Design review of the part built by this model. Coordinates are the model's own, in mm. Face numbers are marked on the shaded views. A direction names the side the tool comes from. Coordinates: 2 decimals unless noted, no trailing zeros. Write each loop counter-clockwise with the first axis right and the second up, starting at its lowest first coordinate (ties: lowest second). Pieces come first, ordered by that corner, then holes. Notation, with made-up numbers: (78.25, 5.5) - (100.25, 5.5) arc R13 ccw to (100.25, 14.5) - close; hole circle Ø8 at (80.25, 83.25). An arc over 180 degrees is marked (long way). Answer as a JSON object with one key per item and string values.
```python
from build123d import *

# Parameters (mm, degrees)
SKETCH1_R           = 6.65
BOSS_EXTRUDE1_DEPTH = 30
SKETCH2_W           = 8
SKETCH2_H           = 40
CUT_EXTRUDE1_DEPTH  = 70.462219947
FILLET1_R           = 4


with BuildPart() as part:
    # Sketch1 → Boss-Extrude1 (new body)
    with BuildSketch(Plane.XY):
        with BuildLine():
            Line((0, 0), (30, 0))
            Line((30, 0), (30, 40))
            ThreePointArc((30, 40), (15, 55), (0, 40))
            Line((0, 40), (0, 0))
        make_face()
        with Locations((15, 40)):
            Circle(SKETCH1_R, mode=Mode.SUBTRACT)
    extrude(amount=BOSS_EXTRUDE1_DEPTH)

    # Sketch2 → Cut-Extrude1 (cut, through all)
    with BuildSketch(Plane.ZY):
        with Locations((15, 35)):
            Rectangle(SKETCH2_W, SKETCH2_H)
    extrude(amount=-CUT_EXTRUDE1_DEPTH, mode=Mode.SUBTRACT)

    # Fillet1
    fillet1_edges = [part.edges().sort_by_distance(p)[0] for p in [
        (15, 15, 19),
        (15, 15, 11),
    ]]
    fillet(fillet1_edges, radius=FILLET1_R - 0.0001)  # a hair under: the kernel refuses the full size


solid = part.part
```
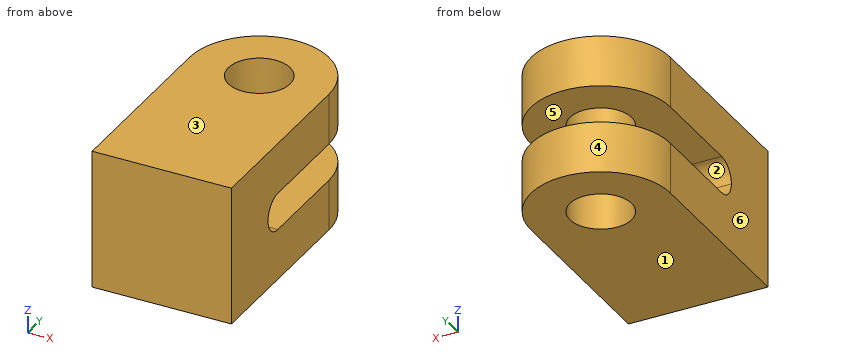
(1) For pin 1 (1 mm diameter, centred on x = 6, z = 24.5, fed in from +Y), flat-tipped, find the tip position at first contact; note if it passes through.
Solved:
{"pin 1": "stops at y = 52.36"}
(2) Take a section at A-A, the plane x = 15. Give the number of separate pieces and of enclosed holes in the cut face, and give its area (3 significant figures).
Solved:
{"separate pieces": "3", "enclosed holes": "0", "area": "1,040 mm^2"}
(3) Take a section at B-B, the plane y = 29.5. Write out the cut boundary in (x, z), and give its area (3 significant figures).
Solved:
{"outline": "(0, 0) - (30, 0) - (30, 11) - (0, 11) - close; (0, 19) - (30, 19) - (30, 30) - (0, 30) - close", "area": "660 mm^2"}
(4) Take a section at D-D, the plane y = 45. Write out the cut boundary in (x, z).
Solved:
{"outline": "(0.86, 0) - (10.62, 0) - (10.62, 11) - (0.86, 11) - close; (0.86, 19) - (10.62, 19) - (10.62, 30) - (0.86, 30) - close; (19.38, 0) - (29.14, 0) - (29.14, 11) - (19.38, 11) - close; (19.38, 19) - (29.14, 19) - (29.14, 30) - (19.38, 30) - close"}
(5) To check wall thickness, follow line 1 (Y direction, x = 15, z = 22.75); line 2 (Z direction, x = 16.75, y = 25.5); line 3 (X direction, y = 40, z = 3). State the ranges of each line that lie inside material, in increasing order. Write a range as from..to.
Solved:
{"line 1": "y = 0..33.35, 46.65..55", "line 2": "z = 0..11, 19..30", "line 3": "x = 0..8.35, 21.65..30"}
(6) Take a section at C-C, the plane z = 8. Write out the cut boundary in (x, y), and give its area (3 significant figures).
Solved:
{"outline": "(0, 0) - (30, 0) - (30, 40) arc R15 ccw to (0, 40) - close; hole circle Ø13.3 at (15, 40)", "area": "1,410 mm^2"}
(7) Tool access review of the marked faces 5 and 6: name each direction out of +Z, -Z, +X, -X, +Y, -Y from which nothing blocks a thin tool from reaching the whole face with its end or side.
Solved:
{"face 5": "+X, -X, +Y", "face 6": "+Z, -Z, -X, +Y, -Y"}
(8) The part is to be moulded in two halves that separate along Z. For the marked faces 1, 2, 3 and 4, say which applies: pulls with the +Z half, pulls with the -Z half, needs draft (parallel to the pull), parting line crosses it, or undercut.
Solved:
{"face 1": "pulls with the -Z half", "face 2": "undercut", "face 3": "pulls with the +Z half", "face 4": "needs draft"}
